from build123d import *

# Parameters (mm, degrees)
F0_R     = 10.5
F0_R_2   = 6
F1_DEPTH = 15
F2_DEPTH = 10.5
F3_R     = 2.5
F4_DEPTH = 12


with BuildPart() as f1:
    # F0 (on Front) → F1 (new body, symmetric)
    with BuildSketch(Plane.XZ):
        Circle(F0_R)
        Circle(F0_R_2, mode=Mode.SUBTRACT)
    extrude(amount=F1_DEPTH, both=True)

    # F0 (on Front) → F2 (join, symmetric)
    with BuildSketch(Plane.XZ):
        Polygon((21, 15), (0, 15), (-21, 15), (-21, -9), (-13, -9), (-10.1991698472, -13), (10.1991698472, -13), (13, -9), (21, -9), align=None)
        Circle(F0_R, mode=Mode.SUBTRACT)
    extrude(amount=F2_DEPTH, both=True)

    # F3 (on face) → F4 (cut)
    with BuildSketch(Plane.XY.offset(15)):
        with Locations((-15.25, 0)):
            Circle(F3_R)
        with Locations((15.25, 0)):
            Circle(F3_R)
    extrude(amount=-F4_DEPTH, mode=Mode.SUBTRACT)


solid = f1.part
Source: CAD feature listing. Evaluate the final solid. Frame: model axes, mm. A direction names the side the tool comes from. Give positions to 0.01 mm unless a question says otherwise; leave off trailing zeros. Write each loop counter-clockwise with the first axis right and the second up, starting at its lowest first coordinate (ties: lowest second). Pieces come first, ordered by that corner, then holes. Notation, with made-up numbers: (58, 47) - (83, 47) arc R21 cw to (83, 76) - close; hole circle Ø1 at (65.5, 81). An arc over 180 degrees is marked (long way). Write item = value, one per line. Start each with the question number.
Q1. Cut plane B-B, the plane x = 0. Return loops of the section in (y, z), then the cut area to 3 significant figures.
Q2. Cut plane D-D, the plane z = 9.25. Return loops of the section in (x, y).
Q3. Cut plane A-A, the plane z = 0. Return loops of the section in (x, y), then the cut area to 3 significant figures.
Q4. Draft query along Y for faces 1 (the cylindrical face through (-6, 0, 0)), 2 (the flat face through (-15, 0, 3)), 3 (the flat face through (0, 10.5, 11)), 4 (the cylindrical face through (-17.748, 0.11, 9.084)). Return one class per face: +Y half, -Y half, draft (parallel to the pull), parting line (faces both ways), or undercut.
Q5. Material intervals for probe 1 along Z at (x, y) = (0, 6.25); probe 2 along Y at (x, z) = (15.25, 10); probe 3 along Y at (x, z) = (12, -5), sorted ascending.
Q6. Pin query (flat end, axial travel): pin 1 Ø1.5 at (x, z) = (-4, 0.5) entering from -Y; pin 2 Ø6.5 at (x, y) = (15.25, 0) entering from -Z; pin 3 Ø3 at (x, z) = (-12.5, -6) entering from -Y; pin 4 Ø5.5 at (x, y) = (-16.5, -1) entering from +Z. Return the tip coordinate at first contact, or that it passes through.
Q7. Reachability of faces 5 (the flat face through (15, 0, 3)), 6 (the cylindrical face through (10, 12.7, 3.2)), 7 (the flat face through (17, 0, -9)), 8 (the flat face through (0, -10.5, 11)) from +Z, -Z, +X, -X, +Y, -Y: full face, straight path, thin tool, end or side. Return the list, or none.
Q8. Cut plane C-C, the plane y = -3.75. Return loops of the section in (x, z).
Computed values:
q1.outline = (-15, -10.5) - (-10.5, -10.5) - (-10.5, -13) - (10.5, -13) - (10.5, -10.5) - (15, -10.5) - (15, -6) - (-15, -6) - close; (-15, 6) - (15, 6) - (15, 10.5) - (10.5, 10.5) - (10.5, 15) - (-10.5, 15) - (-10.5, 10.5) - (-15, 10.5) - close
q1.area = 417 mm²
q2.outline = (-21, -10.5) - (-4.97, -10.5) - (-4.97, -15) - (4.97, -15) - (4.97, -10.5) - (21, -10.5) - (21, 10.5) - (4.97, 10.5) - (4.97, 15) - (-4.97, 15) - (-4.97, 10.5) - (-21, 10.5) - close; hole circle Ø5 at (-15.25, 0); hole circle Ø5 at (15.25, 0)
q3.outline = (-21, -10.5) - (-10.5, -10.5) - (-10.5, -15) - (-6, -15) - (-6, 15) - (-10.5, 15) - (-10.5, 10.5) - (-21, 10.5) - close; (6, -15) - (10.5, -15) - (10.5, -10.5) - (21, -10.5) - (21, 10.5) - (10.5, 10.5) - (10.5, 15) - (6, 15) - close
q3.area = 711 mm²
q4.face_1 = draft
q4.face_2 = undercut
q4.face_3 = +Y half
q4.face_4 = undercut
q5.probe_1 = -13 to -6, 6 to 15
q5.probe_2 = -10.5 to -2.5, 2.5 to 10.5
q5.probe_3 = -10.5 to 10.5
q6.pin_1 = through
q6.pin_2 = -10.43
q6.pin_3 = -10.5
q6.pin_4 = 15
q7.face_5 = +Z
q7.face_6 = +Y
q7.face_7 = -Z, +X, +Y, -Y
q7.face_8 = -Y
q8.outline = (-21, -9) - (-13, -9) - (-10.2, -13) - (10.2, -13) - (13, -9) - (21, -9) - (21, 15) - (-21, 15) - close; hole circle Ø12 at (0, 0)
